For this review, take the finished solid that the model builds, in its own axes (mm). A direction names the side the tool comes from. Coordinates: 2 decimals unless noted, no trailing zeros. Loops run counter-clockwise (first coordinate to the right, second up) from the corner with the lowest first, then second, coordinate; pieces in that order, holes last. Notation, with made-up numbers: (88.5, 41.5) - (99.5, 41.5) arc R14 cw to (99.5, 66.5) - close; hole circle Ø11 at (-0.75, 49.25). An arc over 180 degrees is marked (long way). Use one line per item in the form item = value. Start each with the question number.
1. Add section C-C on x = -12.5. Give the boundary of the cut face in (y, z).
2. Machinability: for faces 1 (the face through (-82, 20.471, 13)), 2 (the face through (1, 19.035, 12)), 3 (the face through (-91.34, 44.02, 25.25)), which of the approach directions +Z, -Z, +X, -X, +Y, -Y give a long, thin tool a straight path to every point of the face, cutting with its end or side? Answer none if there is none.
3. To check wall thickness, follow probe 1 along X at (y, z) = (12, 12.5); probe 2 along Y at (x, z) = (8.5, 15.75); probe 3 along Y at (x, z) = (-63, 22.25). State the ranges of each line that lie inside material, in increasing order.
4. Add section A-A on x = -68. Give the boundary of the cut face in (y, z).
5. Add section B-B on z = 15.5. Give the boundary of the cut face in (x, y), and give its area (3 significant figures).
6. For pin 1 Ø6 at (y, z) = (33.5, 5) entering from -X; pin 2 Ø1 at (y, z) = (22.5, 18) entering from +X; pin 3 Ø7.5 at (y, z) = (45, 10) entering from +X; pin 4 Ø1 at (x, y) = (-80, 11.5) entering from +Z, all flat-tipped, find the tip position at first contact; note any pin that passes through.
```python
from build123d import *

# Parameters (mm, degrees)
F0_R     = 7.733721
F1_DEPTH = 25.4
F2_R     = 2
F3_R     = 0.5


with BuildPart() as f1:
    # F0 (on Top) → F1 (new body)
    with BuildSketch(Plane.XY):
        with BuildLine():
            Line((-110.162757, 0), (0, 0))
            Line((0, 0), (26.410511, 0))
            Line((26.410511, 0), (26.410511, 19.034607))
            Line((26.410511, 19.034607), (-24.819163, 19.034607))
            ThreePointArc((-24.819163, 19.034607), (-29.309291, 20.894479), (-31.169163, 25.384607))
            Line((-31.169163, 25.384607), (-31.169163, 63.743327))
            Line((-31.169163, 63.743327), (-71.819431, 63.743327))
            Line((-71.819431, 63.743327), (-110.162757, 25.4))
            Line((-110.162757, 25.4), (-110.162757, 0))
        make_face()
        with BuildLine():
            ThreePointArc((-98.943353, 18.6625), (-98.41362, 19.941388), (-97.134733, 20.47112))
            Line((-97.134733, 20.47112), (-66.135831, 20.47112))
            Line((-66.135831, 20.47112), (-66.135831, 9.535279))
            Line((-66.135831, 9.535279), (-98.943353, 9.535279))
            Line((-98.943353, 9.535279), (-98.943353, 18.6625))
        make_face(mode=Mode.SUBTRACT)
        with Locations((-58.564864, 38.641442)):
            Circle(F0_R, mode=Mode.SUBTRACT)
    extrude(amount=F1_DEPTH)

    # F2
    f2_edges = [f1.edges().sort_by_distance(p)[0] for p in [
        (-31.169163, 63.743327, 12.7),
    ]]
    fillet(f2_edges, radius=F2_R)

    # F3
    f3_edges = [f1.edges().sort_by_distance(p)[0] for p in [
        (-90.991094, 44.571663, 25.4),
        (-52.494297, 63.743327, 25.4),
    ]]
    fillet(f3_edges, radius=F3_R)


solid = f1.part
```
Conclusion:
q1.outline = (0, 0) - (19.03, 0) - (19.03, 24.9) arc R0.5 ccw to (18.53, 25.4) - (0, 25.4) - close
q2.face_1 = +Z, -Z
q2.face_2 = +Z, -Z, +X, +Y
q2.face_3 = +Z, -X, +Y
q3.probe_1 = -110.16 to -98.94, -66.14 to 26.41
q3.probe_2 = 0 to 19.03
q3.probe_3 = 0 to 32.31, 44.98 to 63.74
q4.outline = (0, 0) - (9.54, 0) - (9.54, 25.4) - (0, 25.4) - close; (20.47, 0) - (63.74, 0) - (63.74, 24.9) arc R0.5 ccw to (63.24, 25.4) - (20.47, 25.4) - close
q5.outline = (-110.16, 0) - (26.41, 0) - (26.41, 19.03) - (-24.82, 19.03) arc R6.35 cw to (-31.17, 25.38) - (-31.17, 61.74) arc R2 ccw to (-33.17, 63.74) - (-71.82, 63.74) - (-110.16, 25.4) - close; hole (-98.94, 9.54) - (-66.14, 9.54) - (-66.14, 20.47) - (-97.13, 20.47) arc R1.81 ccw to (-98.94, 18.66) - close; hole circle Ø15.47 at (-58.56, 38.64)
q5.area = 4,860 mm^2
q6.pin_1 = -105.06
q6.pin_2 = -30.19
q6.pin_3 = -31.17
q6.pin_4 = through
